```python
from build123d import *

# Parameters (mm, degrees)
SKETCH1_R           = 1.75
SKETCH1_W           = 9
SKETCH1_H           = 14
SKETCH1_W_2         = 10
SKETCH1_H_2         = 4
BOSS_EXTRUDE1_DEPTH = 5
FILLET3_R           = 0.5
SKETCH2_R           = 2.85
CUT_EXTRUDE1_DEPTH  = 3.2
SKETCH3_R           = 2.407181936
SKETCH3_R_2         = 2.340327513
SKETCH3_R_3         = 2.41187395
SKETCH3_R_4         = 2.413205516
BOSS_EXTRUDE2_DEPTH = 0.2
SKETCH4_W           = 35
SKETCH4_H           = 35
CUT_EXTRUDE2_DEPTH  = 4
SKETCH5_W           = 9
SKETCH5_H           = 14
BOSS_EXTRUDE3_DEPTH = 1
FILLET2_R           = 1
FILLET1_R           = 2
CHAMFER1_SIZE       = 0.3


with BuildPart() as part:
    # Sketch1 → Boss-Extrude1 (new body)
    with BuildSketch(Plane.XY):
        with BuildLine():
            Line((19.188334778, 20.15), (20.15, 19.188334778))
            Line((20.15, 19.188334778), (20.15, 4.3))
            Line((20.15, 4.3), (23.5, 4.3))
            ThreePointArc((23.5, 4.3), (27.8, 0), (23.5, -4.3))
            Line((23.5, -4.3), (20.15, -4.3))
            Line((20.15, -4.3), (20.15, -19.188334778))
            Line((20.15, -19.188334778), (19.188334778, -20.15))
            Line((19.188334778, -20.15), (4.3, -20.15))
            Line((4.3, -20.15), (4.3, -23.5))
            ThreePointArc((4.3, -23.5), (0, -27.8), (-4.3, -23.5))
            Line((-4.3, -23.5), (-4.3, -20.15))
            Line((-4.3, -20.15), (-19.188334778, -20.15))
            Line((-19.188334778, -20.15), (-20.15, -19.188334778))
            Line((-20.15, -19.188334778), (-20.15, -4.3))
            Line((-20.15, -4.3), (-23.5, -4.3))
            ThreePointArc((-23.5, -4.3), (-27.8, 0), (-23.5, 4.3))
            Line((-23.5, 4.3), (-20.15, 4.3))
            Line((-20.15, 4.3), (-20.15, 19.188334778))
            Line((-20.15, 19.188334778), (-19.188334778, 20.15))
            Line((-19.188334778, 20.15), (-4.3, 20.15))
            Line((-4.3, 20.15), (-4.3, 23.5))
            ThreePointArc((-4.3, 23.5), (0, 27.8), (4.3, 23.5))
            Line((4.3, 23.5), (4.3, 20.15))
            Line((4.3, 20.15), (19.188334778, 20.15))
        make_face()
        with Locations((0, 23.5)):
            Circle(SKETCH1_R, mode=Mode.SUBTRACT)
        with Locations((23.5, 0)):
            Circle(SKETCH1_R, mode=Mode.SUBTRACT)
        with Locations((0, -23.5)):
            Circle(SKETCH1_R, mode=Mode.SUBTRACT)
        with Locations((-23.5, 0)):
            Circle(SKETCH1_R, mode=Mode.SUBTRACT)
        with Locations((10.65, 3.15)):
            Rectangle(SKETCH1_W, SKETCH1_H, mode=Mode.SUBTRACT)
        with Locations((0, -4.5)):
            Rectangle(SKETCH1_W_2, SKETCH1_H_2, mode=Mode.SUBTRACT)
    extrude(amount=BOSS_EXTRUDE1_DEPTH)

    # Fillet3
    fillet3_edges = [part.edges().sort_by_distance(p)[0] for p in [
        (-5, -2.5, 2.5),
        (-5, -6.5, 2.5),
        (5, -6.5, 2.5),
        (5, -2.5, 2.5),
    ]]
    fillet(fillet3_edges, radius=FILLET3_R)

    # Sketch2 → Cut-Extrude1 (cut)
    with BuildSketch(Plane.XY.offset(5)):
        with Locations((0, 23.5)):
            Circle(SKETCH2_R)
        with Locations((23.5, 0)):
            Circle(SKETCH2_R)
        with Locations((-23.5, 0)):
            Circle(SKETCH2_R)
        with Locations((0, -23.5)):
            Circle(SKETCH2_R)
    extrude(amount=-CUT_EXTRUDE1_DEPTH, mode=Mode.SUBTRACT)

    # Sketch3 → Boss-Extrude2 (add)
    with BuildSketch(Plane.XY.offset(1.8)):
        with Locations((0, 23.5)):
            Circle(SKETCH3_R)
        with Locations((23.5, 0)):
            Circle(SKETCH3_R_2)
        with Locations((0, -23.5)):
            Circle(SKETCH3_R_3)
        with Locations((-23.5, 0)):
            Circle(SKETCH3_R_4)
    extrude(amount=-BOSS_EXTRUDE2_DEPTH)

    # Sketch4 → Cut-Extrude2 (cut)
    with BuildSketch(Plane(origin=(0, 0, 0), x_dir=(-1, 0, 0), z_dir=(0, 0, -1))):
        Rectangle(SKETCH4_W, SKETCH4_H)
    extrude(amount=-CUT_EXTRUDE2_DEPTH, mode=Mode.SUBTRACT)

    # Sketch5 → Boss-Extrude3 (add)
    with BuildSketch(Plane(origin=(0, 0, 4), x_dir=(-1, 0, 0), z_dir=(0, 0, -1))):
        Polygon((-16.15, 11.15), (-5.15, 11.15), (-5.15, -1.5), (6, -1.5), (6, -7.5), (-6, -7.5), (-6, -4.85), (-16.15, -4.85), align=None)
        with Locations((-10.65, 3.15)):
            Rectangle(SKETCH5_W, SKETCH5_H, mode=Mode.SUBTRACT)
        with BuildLine():
            Line((5, -3), (5, -6))
            ThreePointArc((5, -6), (4.853553391, -6.353553391), (4.5, -6.5))
            Line((4.5, -6.5), (-4.5, -6.5))
            ThreePointArc((-4.5, -6.5), (-4.853553391, -6.353553391), (-5, -6))
            Line((-5, -6), (-5, -3))
            ThreePointArc((-5, -3), (-4.853553391, -2.646446609), (-4.5, -2.5))
            Line((-4.5, -2.5), (4.5, -2.5))
            ThreePointArc((4.5, -2.5), (4.853553391, -2.646446609), (5, -3))
        make_face(mode=Mode.SUBTRACT)
    extrude(amount=BOSS_EXTRUDE3_DEPTH)

    # Fillet2
    fillet2_edges = [part.edges().sort_by_distance(p)[0] for p in [
        (20.15, 4.3, 2.5),
        (20.15, -4.3, 2.5),
        (4.3, -20.15, 2.5),
        (-4.3, -20.15, 2.5),
        (-20.15, -4.3, 2.5),
        (-20.15, 4.3, 2.5),
        (-4.3, 20.15, 2.5),
        (4.3, 20.15, 2.5),
    ]]
    fillet(fillet2_edges, radius=FILLET2_R)

    # Fillet1
    fillet1_edges = [part.edges().sort_by_distance(p)[0] for p in [
        (-17.5, 17.5, 2),
        (-17.5, -17.5, 2),
        (17.5, -17.5, 2),
        (17.5, 17.5, 2),
    ]]
    fillet(fillet1_edges, radius=FILLET1_R)

    # Chamfer1
    chamfer1_edges = [part.edges().sort_by_distance(p)[0] for p in [
        (0, 27.8, 5),
        (-2.85, 23.5, 5),
        (20.65, 0, 5),
        (-26.35, 0, 5),
        (-2.85, -23.5, 5),
        (-4.3, 22.325, 5),
        (19.669167389, 19.669167389, 0),
        (22.325, 4.3, 0),
        (27.8, 0, 0),
        (-19.669167389, 19.669167389, 5),
        (20.15, -12.244167389, 0),
        (19.669167389, -19.669167389, 0),
        (4.3, -22.325, 0),
        (0, -27.8, 0),
        (-12.244167389, -20.15, 0),
        (-19.669167389, -19.669167389, 0),
        (-22.325, -4.3, 0),
        (-20.15, 12.244167389, 5),
        (-27.8, 0, 0),
        (-20.15, -12.244167389, 0),
        (-20.15, -12.244167389, 5),
        (-22.325, 4.3, 0),
        (-22.325, 4.3, 5),
        (-20.15, 12.244167389, 0),
        (-12.244167389, 20.15, 0),
        (-12.244167389, 20.15, 5),
        (4.3, 22.325, 0),
        (-19.669167389, 19.669167389, 0),
        (4.3, 22.325, 5),
        (20.15, 12.244167389, 0),
        (20.15, 12.244167389, 5),
        (22.325, -4.3, 0),
        (22.325, -4.3, 5),
        (12.244167389, -20.15, 0),
        (12.244167389, -20.15, 5),
        (-4.3, 22.325, 0),
        (-4.3, -22.325, 0),
        (-4.3, -22.325, 5),
        (-20.442893219, -4.592893219, 0),
        (0, 27.8, 0),
        (-20.442893219, -4.592893219, 5),
        (-20.442893219, 4.592893219, 0),
        (-20.442893219, 4.592893219, 5),
        (-4.592893219, 20.442893219, 0),
        (-4.592893219, 20.442893219, 5),
        (4.592893219, 20.442893219, 0),
        (4.592893219, 20.442893219, 5),
        (20.442893219, 4.592893219, 0),
        (20.442893219, 4.592893219, 5),
        (20.442893219, -4.592893219, 0),
        (20.442893219, -4.592893219, 5),
        (4.592893219, -20.442893219, 0),
        (4.592893219, -20.442893219, 5),
        (-4.592893219, -20.442893219, 0),
        (-4.592893219, -20.442893219, 5),
        (12.244167389, 20.15, 0),
        (-17.5, 0, 0),
        (0, -17.5, 0),
        (17.5, 0, 0),
        (0, 17.5, 0),
        (-16.914213562, -16.914213562, 0),
        (16.914213562, -16.914213562, 0),
        (16.914213562, 16.914213562, 0),
        (-16.914213562, 16.914213562, 0),
        (-27.8, 0, 5),
        (-22.325, -4.3, 5),
        (-19.669167389, -19.669167389, 5),
        (12.244167389, 20.15, 5),
        (-12.244167389, -20.15, 5),
        (-1.75, 23.5, 0),
        (0, -27.8, 5),
        (21.75, 0, 0),
        (4.3, -22.325, 5),
        (-1.75, -23.5, 0),
        (-25.25, 0, 0),
        (19.669167389, -19.669167389, 5),
        (20.15, -12.244167389, 5),
        (27.8, 0, 5),
        (22.325, 4.3, 5),
        (19.669167389, 19.669167389, 5),
    ]]
    chamfer(chamfer1_edges, length=CHAMFER1_SIZE)


solid = part.part
```
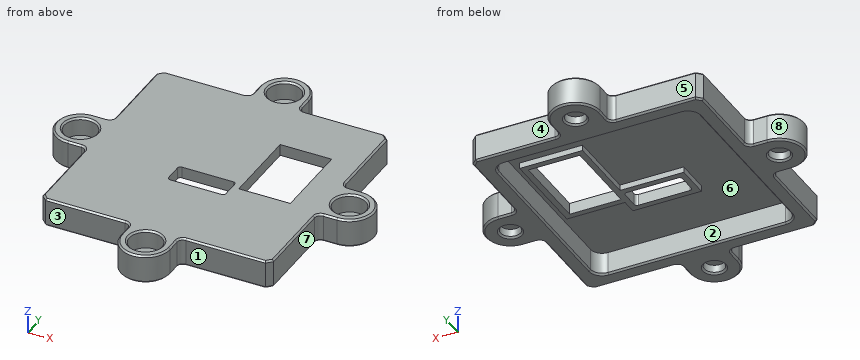
The model under review builds one solid part; all positions refer to its coordinate system, in mm. Face numbers are marked on the shaded views. A direction names the side the tool comes from. Round coordinates to 2 decimals unless told otherwise and drop trailing zeros. Write each loop counter-clockwise with the first axis right and the second up, starting at its lowest first coordinate (ties: lowest second). Pieces come first, ordered by that corner, then holes.
(1) We need section A-A on x = -9. Give the boundary of the cut face in (y, z), and give its area (3 significant figures).
(2) Machinability: for the marked faces 1, 2, 3, 4 and 5, which of the approach directions +Z, -Z, +X, -X, +Y, -Y give a long, thin tool a straight path to every point of the face, cutting with its end or side? Answer none if there is none.
(3) Wall thickness on L1, parallel to Y at x = 0, z = 4.15; L2, parallel to X at y = 0, z = 0.8; L3, parallel to Y at x = -23.5, z = 0.7: over which ranges is each line inside the solid? List them lowest first.
(4) Insertion check: pin 1 (1.1 mm diameter, centred on y = -4.5, z = 3.5, fed in from -X); pin 2 (1.2 mm diameter, centred on y = 22, z = 2, fed in from -X); pin 3 (1 mm diameter, centred on x = 23.5, y = -0.5, fed in from -Z). Each pin has a flat end and moves straight along its axis. Give the tip position at first contact, or say it passes through.
(5) Mouldability with a two-part tool opening along Y and no side actions: class the marked faces 6, 7 and 8 as +Y half, -Y half, draft (parallel to the pull), parting line (faces both ways), or undercut.
Findings below:
1. outline: (-20.15, 0.3) - (-19.85, 0) - (-17.8, 0) - (-17.5, 0.3) - (-17.5, 4) - (17.5, 4) - (17.5, 0.3) - (17.8, 0) - (19.85, 0) - (20.15, 0.3) - (20.15, 4.7) - (19.85, 5) - (-19.85, 5) - (-20.15, 4.7) - close
1. area: 61.2 mm2
2. face 1: +Z, -Z, +X, -Y
2. face 2: -Z
2. face 3: +Z, -Z, -X, -Y
2. face 4: +Z, -Z, +X, +Y
2. face 5: +Z, -Z, -X, +Y
3. L1: y = -27.8 to -26.35, -20.65 to -6.5, -2.5 to 20.65, 26.35 to 27.8
3. L2: x = -27.8 to -25.25, -21.75 to -17.5, 17.5 to 21.75, 25.25 to 27.8
3. L3: y = -4.3 to -1.75, 1.75 to 4.3
4. pin 1: stops at x = -25.2
4. pin 2: stops at x = -4.3
4. pin 3: stops at z = 1.6
5. face 6: undercut
5. face 7: draft
5. face 8: parting line
